Could you check a few things on this model? Use its own coordinates, in mm. A direction names the side the tool comes from. Coordinates: 2 decimals unless noted, no trailing zeros. Write each loop counter-clockwise with the first axis right and the second up, starting at its lowest first coordinate (ties: lowest second). Pieces come first, ordered by that corner, then holes.
```python
from build123d import *

# Parameters (mm, degrees)
SKETCH1_W           = 120
SKETCH1_H           = 120
SKETCH1_R           = 7.5
BOSS_EXTRUDE1_DEPTH = 10
BOSS_EXTRUDE2_DEPTH = 200
SKETCH2_R           = 3.25
CUT_EXTRUDE1_DEPTH  = 15


with BuildPart() as part:
    # Sketch1 → Boss-Extrude1 (new body)
    with BuildSketch(Plane(origin=(0, 0, 0), x_dir=(1, 0, 0), z_dir=(0, 1, 0))):
        with Locations((60, 60)):
            Rectangle(SKETCH1_W, SKETCH1_H)
        with Locations(Location((60, 60, 0), (0, 0, 270))):
            Circle(SKETCH1_R, mode=Mode.SUBTRACT)
    extrude(amount=BOSS_EXTRUDE1_DEPTH)

    # 3DSketch1 → Boss-Extrude2 (add)
    with BuildSketch(Plane(origin=(110, 10, -10), x_dir=(-0.7071067811865477, 0, -0.7071067811865475), z_dir=(0, 1, 0))):
        Polygon((155.563491861, 0), (70.710678119, 84.852813742), (-14.142135624, 0), (70.710678119, -84.852813742), align=None)
        Polygon((0, 0), (70.710678119, -70.710678119), (141.421356237, 0), (70.710678119, 70.710678119), align=None, mode=Mode.SUBTRACT)
    extrude(amount=BOSS_EXTRUDE2_DEPTH)

    # Sketch2 → Cut-Extrude1 (cut)
    with BuildSketch(Plane(origin=(0, 210, 0), x_dir=(1, 0, 0), z_dir=(0, 1, 0))):
        with Locations(Location((115, 115, 0), (0, 0, 270))):
            Circle(SKETCH2_R)
        with Locations(Location((5, 115, 0), (0, 0, 270))):
            Circle(SKETCH2_R)
        with Locations(Location((115, 5, 0), (0, 0, 270))):
            Circle(SKETCH2_R)
        with Locations(Location((5, 5, 0), (0, 0, 270))):
            Circle(SKETCH2_R)
    extrude(amount=-CUT_EXTRUDE1_DEPTH, mode=Mode.SUBTRACT)


solid = part.part
```
1. If we mould it in two halves opening along X, with no side actions, what happens to faces 1 (the face through (0, 104, -61)), 2 (the face through (46, 0, -61)), 3 (the face through (10, 109, -61))? For each: pulls with the +X half, pulls with the -X half, needs draft (parallel to the pull), parting line crosses it, or undercut.
Verdict:
face 1: pulls with the -X half
face 2: needs draft
face 3: undercut
2. I want a section at A-A on y = 180. Please give me the cut outline in (x, z).
Verdict:
outline: (0, -120) - (120, -120) - (120, 0) - (0, 0) - close; hole (10, -110) - (110, -110) - (110, -10) - (10, -10) - close
3. I want a section at C-C on x = 60. Please give me the cut outline in (y, z), plus the area to 3 significant figures.
Verdict:
outline: (0, -120) - (210, -120) - (210, -110) - (10, -110) - (10, -67.5) - (0, -67.5) - close; (0, -52.5) - (10, -52.5) - (10, -10) - (210, -10) - (210, 0) - (0, 0) - close
area: 5,050 mm2
4. On a 3-axis mill with a long thin cutter (end or side, diameter ignored), from which of +Z, -Z, +X, -X, +Y, -Y can I reach the whole of each face in a straight line? I mean faces 4 (the face through (65.1, 4.9, -65.5)), 5 (the face through (110, 109, -59)). Say none if no direction works.
Verdict:
face 4: +Y, -Y
face 5: +Y
5. I want a section at D-D on x = 88. Please give me the cut outline in (y, z), plus the area to 3 significant figures.
Verdict:
outline: (0, -120) - (210, -120) - (210, -110) - (10, -110) - (10, -10) - (210, -10) - (210, 0) - (0, 0) - close
area: 5,200 mm2
6. I want a section at B-B on z = -60. Please give me the cut outline in (x, y), plus the area to 3 significant figures.
Verdict:
outline: (0, 0) - (52.5, 0) - (52.5, 10) - (10, 10) - (10, 210) - (0, 210) - close; (67.5, 0) - (120, 0) - (120, 210) - (110, 210) - (110, 10) - (67.5, 10) - close
area: 5,050 mm2
7. Please list where these lines run through material, in increasing order: line 1 along X through (y, z) = (15, -80); line 2 along X through (y, z) = (6, -60); line 3 along Z through (x, y) = (47.5, 87.5).
Verdict:
line 1: x = 0 to 10, 110 to 120
line 2: x = 0 to 52.5, 67.5 to 120
line 3: z = -120 to -110, -10 to 0
8. For pin 1 (9 mm diameter, centred on x = 60, z = -60, fed in from -Y); pin 2 (2 mm diameter, centred on x = 29, z = -105, fed in from +Y); pin 3 (2 mm diameter, centred on x = 6.5, z = -115.5, fed in from +Y), each with a flat end and sliding along its axis, tell me the tip position at first contact or that it passes through.
Verdict:
pin 1: passes through
pin 2: stops at y = 10
pin 3: stops at y = 195
